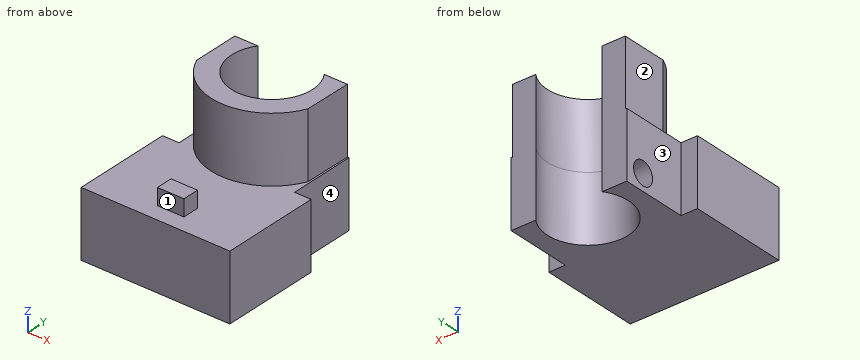
from build123d import *

# Parameters (mm, degrees)
BOSS_EXTRUDE1_DEPTH     = 20
SKETCH2_W               = 8
SKETCH2_H               = 5
BOSS_EXTRUDE2_DEPTH     = 5
SKETCH3_R               = 12.25
CUT_EXTRUDE1_DEPTH      = 20
BOSS_EXTRUDE3_DEPTH     = 20
SKETCH6_R               = 3.5
CUT_EXTRUDE2_DEPTH      = 1
CUT_EXTRUDE2_DEPTH_BACK = 8


with BuildPart() as part:
    # Sketch1 → Boss-Extrude1 (new body)
    with BuildSketch(Plane.XY):
        Polygon((17.5, 15), (22.5, 15), (22.5, -15), (-22.5, -15), (-22.5, 15), (-17.5, 15), (-17.5, 35), (17.5, 35), align=None)
    extrude(amount=BOSS_EXTRUDE1_DEPTH)

    # Sketch2 → Boss-Extrude2 (add)
    with BuildSketch(Plane.XY.offset(20)):
        with Locations((0.5, -7.5)):
            Rectangle(SKETCH2_W, SKETCH2_H)
    extrude(amount=BOSS_EXTRUDE2_DEPTH)

    # Sketch3 → Cut-Extrude1 (cut)
    with BuildSketch(Plane.XY.offset(20)):
        with Locations((0, 28)):
            Circle(SKETCH3_R)
    extrude(amount=-CUT_EXTRUDE1_DEPTH, mode=Mode.SUBTRACT)

    # Sketch4 → Boss-Extrude3 (add)
    with BuildSketch(Plane.XY.offset(20)):
        with BuildLine():
            Line((-17.036725037, 35), (-17.036725037, 21))
            ThreePointArc((-17.036725037, 21), (-0.167488081, 9.582021073), (16.906605879, 20.691328599))
            Line((16.906605879, 20.691328599), (17.036725037, 35))
            Line((17.036725037, 35), (10.052984631, 35))
            ThreePointArc((10.052984631, 35), (0, 15.75), (-10.052984631, 35))
            Line((-10.052984631, 35), (-17.036725037, 35))
        make_face()
    extrude(amount=BOSS_EXTRUDE3_DEPTH)

    # Sketch6 → Cut-Extrude2 (cut, two sides)
    with BuildSketch(Plane.ZY.offset(17.5)) as cut_extrude2_sk:
        with Locations((5, 29)):
            Circle(SKETCH6_R)
    extrude(amount=CUT_EXTRUDE2_DEPTH, mode=Mode.SUBTRACT)
    extrude(cut_extrude2_sk.sketch, amount=-CUT_EXTRUDE2_DEPTH_BACK, mode=Mode.SUBTRACT)


solid = part.part
The model under review builds one solid part; all positions refer to its coordinate system, in mm. Face numbers are marked on the shaded views. A direction names the side the tool comes from. Round coordinates to 2 decimals unless told otherwise and drop trailing zeros. Write each loop counter-clockwise with the first axis right and the second up, starting at its lowest first coordinate (ties: lowest second). Pieces come first, ordered by that corner, then holes. Notation, with made-up numbers: M 76,30 L 103,30 A16 cw 103,48 Z; hole C 69,11.5 d5. An arc over 180 degrees is marked long. Answer as CSV lines item,"result". Start each with the question number.
Q1. Wall thickness on line 1 along X through (y, z) = (28, 14); line 2 along Z through (x, y) = (-13.75, 29); line 3 along Y through (x, z) = (-15.5, 5): over which ranges is each line inside the solid? List them lowest first.
Q2. Tool access review of the marked faces 1, 2, 3 and 4: name each direction out of +Z, -Z, +X, -X, +Y, -Y from which nothing blocks a thin tool from reaching the whole face with its end or side.
Q3. Consider section D-D, the plane z = 30.5. Give the boundary of the cut face in (x, y).
Q4. Consider section C-C, the plane x = 11. Give the boundary of the cut face in (y, z), then the cut area to 3 significant figures.
Q5. Clearance check with flat-ended pins moving along their axes: P1, Ø12, axis at x = 0, z = 15.5, coming from the +Y side; P2, Ø8, axis at y = 29, z = 5, coming from the +X side; P3, Ø2.5, axis at x = 0, z = 22, coming from the +Y side; P4, Ø12, axis at x = 12.5, y = 27.5, coming from the -Z side. State where each tip first meets the part, or that it passes through.
Q6. Consider section B-B, the plane z = 5. Give the boundary of the cut face in (x, y), then the cut area to 3 significant figures.
Q7. Consider section A-A, the plane y = 28. Give the boundary of the cut face in (x, z), then the cut area to 3 significant figures.
Result set:
1,line 1,"x = -17.5 to -12.25, 12.25 to 17.5"
1,line 2,"z = 0 to 1.5, 8.5 to 40"
1,line 3,"y = -15 to 25.5, 32.5 to 35"
2,face 1,"+Z, +X, -X, -Y"
2,face 2,"+Z, -X, +Y, -Y"
2,face 3,"+Z, -Z, -X, +Y"
2,face 4,"+Z, -Z, +X, +Y"
3,outline,"M -17.04,21 A18.42 ccw 16.91,20.69 L 17.04,35 L 10.05,35 A12.25 cw long -10.05,35 L -17.04,35 Z"
4,outline,"M -15,0 L 22.61,0 L 22.61,40 L 13.23,40 L 13.23,20 L -15,20 Z; M 33.39,0 L 35,0 L 35,40 L 33.39,40 Z"
4,area,"1,000 mm²"
5,P1,"stops at y = 17.32"
5,P2,"stops at x = 17.5"
5,P3,"stops at y = 15.81"
5,P4,"stops at z = 0"
6,outline,"M -22.5,-15 L 22.5,-15 L 22.5,15 L 17.5,15 L 17.5,35 L 10.05,35 A12.25 cw long -11.99,25.5 L -17.5,25.5 L -17.5,15 L -22.5,15 Z; M -17.5,32.5 L -11.39,32.5 A12.25 cw -10.05,35 L -17.5,35 Z"
6,area,"1,610 mm²"
7,outline,"M -17.5,0 L -12.25,0 L -12.25,1.65 L -17.5,1.65 Z; M -17.5,8.35 L -12.25,8.35 L -12.25,40 L -17.04,40 L -17.04,20 L -17.5,20 Z; M 12.25,0 L 17.5,0 L 17.5,20 L 16.97,20 L 16.97,40 L 12.25,40 Z"
7,area,"365 mm²"
